Could you check a few things on this drawing? It's one solid part, dimensions in mm from its lowest x, y, z. A direction names the side the tool comes from. Give positions to 0.01 mm unless a question says otherwise; leave off trailing zeros. Order: outer loops, then holes, each group sorted by start corner. A loop starts at its lowest first (then second) coordinate and runs counter-clockwise, first axis right, second up. Notation, with made-up numbers: (7.25, 84) -> (40.25, 84) arc R21 ccw to (40.25, 111) -> close; hole circle Ø1 at (71, 54). An arc over 180 degrees is marked (long way). Write each question's results on one line, items separated by ' | '. Start each with the question number.
Q1. Imagine slicing it at C-C, the plane x = 77. Please give me the cut outline in (y, z), then the cut area to 3 significant figures.
Q2. Imagine slicing it at A-A, the plane y = 55.5. Please give me the cut outline in (x, z), then the cut area to 3 significant figures.
Q3. I need wall thicknesses on line 1 along X through (y, z) = (101, 4); line 2 along Z through (x, y) = (3, 97.5). Which ranges of each line are inside material? Lowest first, please. Write a range as [from, to].
Q4. I'm going to push flat-ended pins straight in: pin 1 (4.5 mm diameter, centred on x = 5, y = 55.5, fed in from +Z); pin 2 (5 mm diameter, centred on y = 61, z = 14, fed in from -X); pin 3 (1.5 mm diameter, centred on y = 38.5, z = 1.5, fed in from +X). Where does each tip first touch, or does it pass through?
Q5. For the marked faces 1, 2, 3 and 4, which set-ups out of +Z, -Z, +X, -X, +Y, -Y let a thin tool reach every point of the face, with its end or its side?
Q6. Imagine slicing it at B-B, the plane z = 3.25. Please give me the cut outline in (x, y).
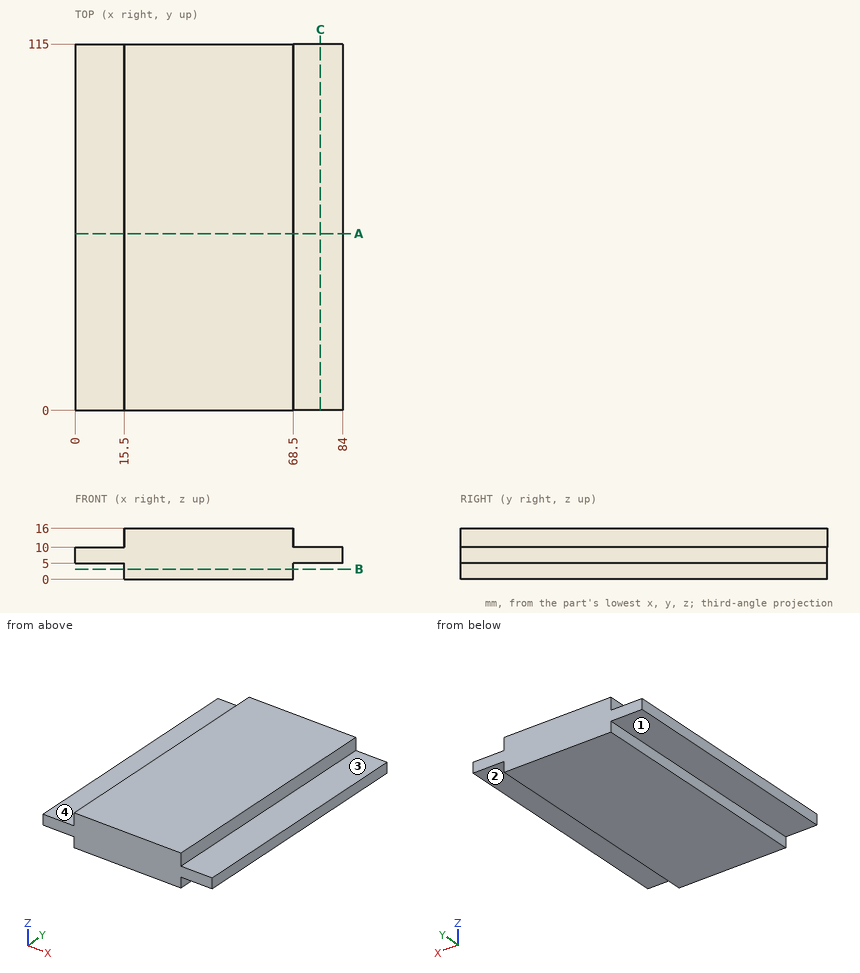
Geometry check:
1) outline: (0, 5) -> (115, 5) -> (115, 10) -> (0, 10) -> close | area: 575 mm²
2) outline: (0, 5) -> (15.5, 5) -> (15.5, 0) -> (68.5, 0) -> (68.5, 5) -> (84, 5) -> (84, 10) -> (68.5, 10) -> (68.5, 16) -> (15.5, 16) -> (15.5, 10) -> (0, 10) -> close | area: 1,000 mm²
3) line 1: [15.5, 68.5] | line 2: [5, 10]
4) pin 1: z = 10 | pin 2: x = 15.5 | pin 3: x = 68.5
5) face 1: -Z, -X, +Y, -Y | face 2: -Z, +X, +Y, -Y | face 3: +Z, +X, +Y, -Y | face 4: +Z, -X, +Y, -Y
6) outline: (15.5, 0) -> (68.5, 0) -> (68.5, 115) -> (15.5, 115) -> close
